```python
from build123d import *

# Parameters (mm, degrees)
SKETCH1_R               = 5.5
BOSS_EXTRUDE1_DEPTH     = 0.94
SKETCH3_R               = 3.78
BOSS_EXTRUDE2_DEPTH     = 1.5
SKETCH4_R               = 4.25
BOSS_EXTRUDE3_DEPTH     = 0.0625
SKETCH5_R               = 3.36
CUT_EXTRUDE1_DEPTH      = 20
CUT_EXTRUDE1_DEPTH_BACK = 6.0625
SKETCH7_R               = 0.44
CUT_EXTRUDE2_DEPTH      = 7.0625
CIRPATTERN1_COUNT       = 8
SCALE1_SCALE            = 25.4


with BuildPart() as part:
    # Sketch1 → Boss-Extrude1 (new body)
    with BuildSketch(Plane(origin=(0, 0, 0), x_dir=(1, 0, 0), z_dir=(0, 1, 0))):
        Circle(SKETCH1_R)
    extrude(amount=BOSS_EXTRUDE1_DEPTH)

    # Sketch3 → Boss-Extrude2 (add)
    with BuildSketch(Plane(origin=(0, 0, 0), x_dir=(1, 0, 0), z_dir=(0, 1, 0))):
        Circle(SKETCH3_R)
    extrude(amount=BOSS_EXTRUDE2_DEPTH)

    # Sketch4 → Boss-Extrude3 (add)
    with BuildSketch(Plane(origin=(0, 0, 0), x_dir=(1, 0, 0), z_dir=(0, 1, 0))):
        Circle(SKETCH4_R)
    extrude(amount=-BOSS_EXTRUDE3_DEPTH)

    # Sketch5 → Cut-Extrude1 (cut, two sides)
    with BuildSketch(Plane(origin=(0, 0, 0), x_dir=(1, 0, 0), z_dir=(0, 1, 0))) as cut_extrude1_sk:
        Circle(SKETCH5_R)
    extrude(amount=CUT_EXTRUDE1_DEPTH, mode=Mode.SUBTRACT)
    extrude(cut_extrude1_sk.sketch, amount=-CUT_EXTRUDE1_DEPTH_BACK, mode=Mode.SUBTRACT)

    # Sketch7 → Cut-Extrude2 (cut)
    with BuildSketch(Plane(origin=(0, 0, 0), x_dir=(1, 0, 0), z_dir=(0, 1, 0))):
        with Locations((0, 4.75)):
            Circle(SKETCH7_R)
    cut_extrude2 = extrude(amount=CUT_EXTRUDE2_DEPTH, mode=Mode.SUBTRACT)

    # CirPattern1: Cut-Extrude2 ×8 about axis
    cirpattern1_axis = Axis((0, 0, 0), (0, 1, 0))
    for i in range(1, CIRPATTERN1_COUNT):
        add(cut_extrude2.rotate(cirpattern1_axis, i * 360 / CIRPATTERN1_COUNT), mode=Mode.SUBTRACT)


with BuildPart() as part_1:
    # Scale1: scaled about (0, 0.526704923, 0)
    add(part.part.scale(SCALE1_SCALE).moved(Location((0, -12.851600121, 0))))


solid = part_1.part
```
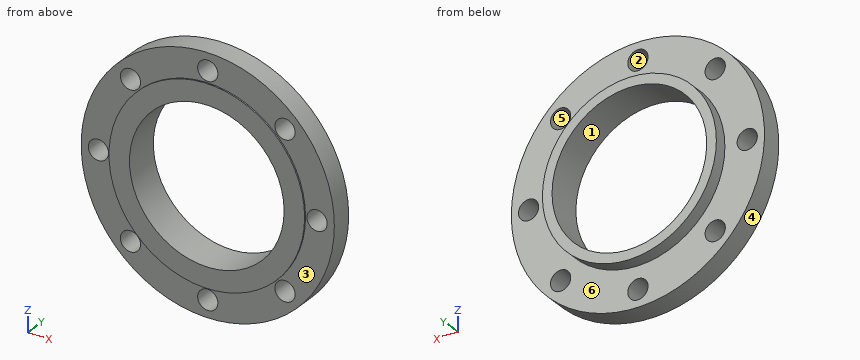
Work out the finished part from the listing and answer in its coordinate system (mm). Face numbers are marked on the shaded views. A direction names the side the tool comes from. Coordinates: 2 decimals unless noted, no trailing zeros. Order: outer loops, then holes, each group sorted by start corner. A loop starts at its lowest first (then second) coordinate and runs counter-clockwise, first axis right, second up. Notation, with made-up numbers: (23, -40) - (63, -40) arc R25 cw to (63, -21) - close; hole circle Ø8 at (-17, -40). An arc over 180 degrees is marked (long way). Answer as a JSON object with one key per item and string values.
1. The mould has two halves that part along Z. Classify the marked faces 1, 2, 3 and 4: +Z half, -Z half, draft (parallel to the pull), parting line (faces both ways), or undercut.
Output values:
{"face 1": "undercut", "face 2": "undercut", "face 3": "draft", "face 4": "parting line"}
2. Find section C-C on z = 120.65. Determine the outline of the cut face in (x, y), plus the area to 3 significant figures.
Output values:
{"outline": "(-70.42, -12.85) - (-11.18, -12.85) - (-11.18, 11.02) - (-70.42, 11.02) - close; (11.18, -12.85) - (70.42, -12.85) - (70.42, 11.02) - (11.18, 11.02) - close", "area": "2,830 mm²"}
3. Find section D-D on y = 5.5. Count the separate pieces of the cut face and the enclosed holes in it, plus the area to 3 significant figures.
Output values:
{"separate pieces": "1", "enclosed holes": "9", "area": "35,300 mm²"}
4. Find section B-B on z = 0. Determine the outline of the cut face in (x, y).
Output values:
{"outline": "(-139.7, -12.85) - (-131.83, -12.85) - (-131.83, 11.02) - (-139.7, 11.02) - close; (-109.47, -12.85) - (-107.95, -12.85) - (-107.95, -14.44) - (-85.34, -14.44) - (-85.34, 25.25) - (-96.01, 25.25) - (-96.01, 11.02) - (-109.47, 11.02) - close; (85.34, -14.44) - (107.95, -14.44) - (107.95, -12.85) - (109.47, -12.85) - (109.47, 11.02) - (96.01, 11.02) - (96.01, 25.25) - (85.34, 25.25) - close; (131.83, -12.85) - (139.7, -12.85) - (139.7, 11.02) - (131.83, 11.02) - close"}
5. Each of these flat-tipped pins is pushed along its axis until it touches: P1, Ø12, axis at y = 2.5, z = -66.5, coming from the +X side; P2, Ø3, axis at x = 45, y = 1, coming from the -Z side; P3, Ø10, axis at x = -38.5, y = 5, coming from the +Z side. Where does it stop, or does it pass through?
Output values:
{"P1": "stops at x = 125.92", "P2": "stops at z = -132.75", "P3": "stops at z = 135.62"}
6. Consider line 1 (X direction, y = 8, z = 0); line 2 (X direction, y = 13, z = 0). Determine where each line is inside the solid, lowest interval first.
Output values:
{"line 1": "x = -139.7 to -131.83, -109.47 to -85.34, 85.34 to 109.47, 131.83 to 139.7", "line 2": "x = -96.01 to -85.34, 85.34 to 96.01"}
7. A tool of negligible diameter and unlimited length cuts with its end or side. For the marked faces 5 and 6, from which of +Z, -Z, +X, -X, +Y, -Y can it reach the whole face along a straight path? Write none if from no direction.
Output values:
{"face 5": "+Y, -Y", "face 6": "+Y"}
8. Find section A-A on x = 0. Determine the outline of the cut face in (y, z), plus the area to 3 significant figures.
Output values:
{"outline": "(-14.44, -107.95) - (-12.85, -107.95) - (-12.85, -109.47) - (11.02, -109.47) - (11.02, -96.01) - (25.25, -96.01) - (25.25, -85.34) - (-14.44, -85.34) - close; (-14.44, 85.34) - (25.25, 85.34) - (25.25, 96.01) - (11.02, 96.01) - (11.02, 109.47) - (-12.85, 109.47) - (-12.85, 107.95) - (-14.44, 107.95) - close; (-12.85, -139.7) - (11.02, -139.7) - (11.02, -131.83) - (-12.85, -131.83) - close; (-12.85, 131.83) - (11.02, 131.83) - (11.02, 139.7) - (-12.85, 139.7) - close", "area": "1,900 mm²"}
